Verification items for the finished model (mm, model axes). A direction names the side the tool comes from. Round coordinates to 2 decimals unless told otherwise and drop trailing zeros. Order: outer loops, then holes, each group sorted by start corner. A loop starts at its lowest first (then second) coordinate and runs counter-clockwise, first axis right, second up. Notation, with made-up numbers: (23, 71) -> (30, 71) arc R22 cw to (30, 107) -> close; hole circle Ø11 at (28, -9). An arc over 180 degrees is marked (long way). Return JSON: item names as keys, results as strings. Group by question number.
1) Section check A-A on x = 28. Enter the section's corners in (y, z) (3 decimals), plus the area to 3 significant figures.
2) Depth check by flat-ended pin: pin 1 (1.6 mm diameter, centred on y = 1, z = -29.5, fed in from +X); pin 2 (2.5 mm diameter, centred on x = 3.48, z = -30.2, fed in from -Y); pin 3 (1 mm diameter, centred on x = 26.5, y = 1.5, fed in from -Z). Enter the tip coordinate at first touch or a pass-through.
3) Section check D-D on x = 37. Enter the section's corners in (y, z) (3 decimals).
4) Draft check along Z on faces 1 (the cylindrical face through (1.45, 1.57, -4.89)), 2 (the flat face through (16.181, 2, -32)), 3 (the flat face through (29, 2, -17.496)). Enter one of: pulls with the +Z half, pulls with the -Z half, needs draft (parallel to the pull), parting line crosses it, or undercut.
5) Scan lines: L1, parallel to X at y = 2.9, z = -4; L2, parallel to Z at x = 5, y = 0.6; L3, parallel to Z at x = 35, y = 1.6. Record each from-to range of solid material in increasing order.
6) Section check C-C on z = -37.5. Enter the section's corners in (x, y) (3 decimals).
7) Section check B-B on y = 1.25. Enter the section's corners in (x, z).
8) Tool access check on faces 4 (the flat face through (-22, 2, -17.496)), 5 (the cylindrical face through (40.82, 1.57, -16.77)). Record the directions out of +Z, -Z, +X, -X, +Y, -Y that give a thin tool (end or side, any length) a straight path to the whole face; none if there is none.
```python
from build123d import *

# Parameters (mm, degrees)
SKETCH1_R           = 2.032
BOSS_EXTRUDE1_DEPTH = 3.175


with BuildPart() as part:
    # Sketch1 → Boss-Extrude1 (new body)
    with BuildSketch(Plane(origin=(0, 0, 0), x_dir=(1, 0, 0), z_dir=(0, 1, 0))):
        with BuildLine():
            Line((18.720543933, 17.495711297), (39.040543933, 17.495711297))
            ThreePointArc((39.040543933, 17.495711297), (40.836595157, 16.751762521), (41.580543933, 14.955711297))
            Line((41.580543933, 14.955711297), (41.580543933, -5.364288703))
            ThreePointArc((41.580543933, -5.364288703), (40.836595157, -7.160339927), (39.040543933, -7.904288703))
            Line((39.040543933, -7.904288703), (-32.079456067, -7.904288703))
            ThreePointArc((-32.079456067, -7.904288703), (-33.875507291, -7.160339927), (-34.619456067, -5.364288703))
            Line((-34.619456067, -5.364288703), (-34.619456067, 14.955711297))
            ThreePointArc((-34.619456067, 14.955711297), (-33.875507291, 16.751762521), (-32.079456067, 17.495711297))
            Line((-32.079456067, 17.495711297), (-11.759456067, 17.495711297))
            ThreePointArc((-11.759456067, 17.495711297), (-9.963404843, 18.239660073), (-9.219456067, 20.035711297))
            Line((-9.219456067, 20.035711297), (-9.219456067, 42.895711297))
            Line((-9.219456067, 42.895711297), (16.180543933, 42.895711297))
            Line((16.180543933, 42.895711297), (16.180543933, 20.035711297))
            ThreePointArc((16.180543933, 20.035711297), (16.924492709, 18.239660073), (18.720543933, 17.495711297))
        make_face()
        with Locations((3.480543933, 4.795711297)):
            Circle(SKETCH1_R, mode=Mode.SUBTRACT)
        with Locations((-21.919456067, 4.795711297)):
            Circle(SKETCH1_R, mode=Mode.SUBTRACT)
        with Locations((28.880543933, 4.795711297)):
            Circle(SKETCH1_R, mode=Mode.SUBTRACT)
        with Locations((3.480543933, 30.195711297)):
            Circle(SKETCH1_R, mode=Mode.SUBTRACT)
    extrude(amount=BOSS_EXTRUDE1_DEPTH)


solid = part.part
```
Check result:
{
 "1": {"outline": "(0, -17.496) -> (3.175, -17.496) -> (3.175, -6.627) -> (0, -6.627) -> close; (0, -2.964) -> (3.175, -2.964) -> (3.175, 7.904) -> (0, 7.904) -> close", "area": "69.0 mm^2"},
 "2": {"pin 1": "x = 16.18", "pin 2": "through", "pin 3": "z = -17.5"},
 "3": {"outline": "(0, -17.496) -> (3.175, -17.496) -> (3.175, 7.904) -> (0, 7.904) -> close"},
 "4": {"face 1": "undercut", "face 2": "needs draft", "face 3": "pulls with the -Z half"},
 "5": {"L1": "-34.62 to -23.79, -20.05 to 1.61, 5.35 to 27.01, 30.75 to 41.58", "L2": "-42.9 to -31.54, -28.85 to -6.14, -3.45 to 7.9", "L3": "-17.5 to 7.9"},
 "6": {"outline": "(-9.219, 0) -> (16.181, 0) -> (16.181, 3.175) -> (-9.219, 3.175) -> close"},
 "7": {"outline": "(-34.62, -14.96) arc R2.54 ccw to (-32.08, -17.5) -> (-11.76, -17.5) arc R2.54 cw to (-9.22, -20.04) -> (-9.22, -42.9) -> (16.18, -42.9) -> (16.18, -20.04) arc R2.54 cw to (18.72, -17.5) -> (39.04, -17.5) arc R2.54 ccw to (41.58, -14.96) -> (41.58, 5.36) arc R2.54 ccw to (39.04, 7.9) -> (-32.08, 7.9) arc R2.54 ccw to (-34.62, 5.36) -> close; hole circle Ø4.06 at (-21.92, -4.8); hole circle Ø4.06 at (3.48, -30.2); hole circle Ø4.06 at (3.48, -4.8); hole circle Ø4.06 at (28.88, -4.8)"},
 "8": {"face 4": "-Z, -X, +Y, -Y", "face 5": "-Z, +X, +Y, -Y"}
}
